from build123d import *

# Parameters (mm, degrees)
F0_W     = 1000
F0_H     = 1000
F1_DEPTH = 500
F2_W     = 940
F2_H     = 940
F3_DEPTH = 10
F4_T     = -1.5


# Not quite as in the source:
# - a shell that OpenCascade refuses in one call is made with other operations: the cavity is built on its own and cut out


with BuildPart() as f1:
    # F0 (on Top) → F1 (new body)
    with BuildSketch(Plane.XY):
        Rectangle(F0_W, F0_H)
    extrude(amount=F1_DEPTH)

    # F2 (on face) → F3 (cut)
    with BuildSketch(Plane(origin=(0, 0, 0), x_dir=(1, 0, 0), z_dir=(0, 0, -1))):
        Rectangle(F2_W, F2_H)
    extrude(amount=-F3_DEPTH, mode=Mode.SUBTRACT)

    # F4: a shell. OpenCascade refuses it in one call, so the cavity is built on its own and cut out:
    # the body offset inwards by the wall thickness, plus a prism from it out through each open face.
    f4_core = offset(f1.part, amount=F4_T, kind=Kind.INTERSECTION, mode=Mode.PRIVATE)
    f4_exits = [f4_core.faces().sort_by_distance(p)[0] for p in [
        (0, 0, 11.5),
    ]]
    add(f4_core, mode=Mode.SUBTRACT)
    extrude(f4_exits, amount=-F4_T, mode=Mode.SUBTRACT)


solid = f1.part
Source: CAD feature listing. Evaluate the final solid. Frame: model axes, mm. A direction names the side the tool comes from. Give positions to 0.01 mm unless a question says otherwise; leave off trailing zeros. Write each loop counter-clockwise with the first axis right and the second up, starting at its lowest first coordinate (ties: lowest second). Pieces come first, ordered by that corner, then holes. Notation, with made-up numbers: M 59,6.25 L 93,6.25 A16 cw 93,13.25 Z; hole C -26.75,-5 d2. An arc over 180 degrees is marked long. Return JSON: item names as keys, results as strings. Group by question number.
1) Cut plane A-A, the plane x = 218.5. Output: boundary loops of the cut face in (y, z), plus the area to 3 significant figures.
2) Cut plane B-B, the plane z = 176.5. Output: boundary loops of the cut face in (x, y).
3) Pull-direction query (Z, two-part tool) for faces 3 (the face through (-7, -500, 246)), 4 (the face through (-39, -479, 0)), 5 (the face through (-39, -478, 1.5)); classes: pulls with the +Z half, pulls with the -Z half, needs draft (parallel to the pull), parting line crosses it, or undercut.
4) Set-up query: faces 1 (the face through (-7, -498.5, 247)), 2 (the face through (500, -7, 246)). Return all of +Z, -Z, +X, -X, +Y, -Y with unobstructed straight access to the full face (end or side cutting, diameter ignored); none if empty.
5) Material intervals for line 1 along X through (y, z) = (446, 325.5); line 2 along Z through (x, y) = (317, 375.5), sorted ascending. Write a range as [from, to].
Recorded:
{
 "1": {"outline": "M -500,0 L -470,0 L -470,10 L -471.5,10 L -471.5,1.5 L -498.5,1.5 L -498.5,498.5 L 498.5,498.5 L 498.5,1.5 L 471.5,1.5 L 471.5,10 L 470,10 L 470,0 L 500,0 L 500,500 L -500,500 Z", "area": "3,110 mm²"},
 "2": {"outline": "M -500,-500 L 500,-500 L 500,500 L -500,500 Z; hole M -498.5,-498.5 L 498.5,-498.5 L 498.5,498.5 L -498.5,498.5 Z"},
 "3": {"face 3": "needs draft", "face 4": "pulls with the -Z half", "face 5": "undercut"},
 "4": {"face 1": "none", "face 2": "+Z, -Z, +X, +Y, -Y"},
 "5": {"line 1": "x = [-500, -498.5], [498.5, 500]", "line 2": "z = [498.5, 500]"}
}
